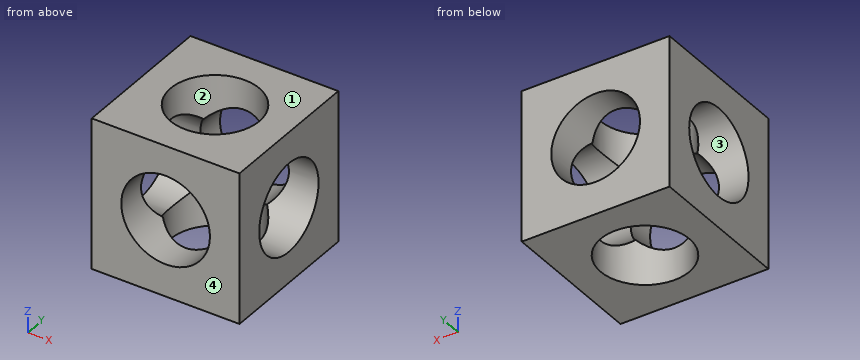
```python
from build123d import *

# Parameters (mm, degrees)
F0_W     = 126.93037
F0_H     = 126.93037
F0_R     = 38.1
F1_DEPTH = 129.5146
F2_R     = 38.1
F3_DEPTH = 129.5146
F4_R     = 38.1
F5_DEPTH = 129.5146


with BuildPart() as f1:
    # F0 (on Top) → F1 (new body)
    with BuildSketch(Plane.XY):
        Rectangle(F0_W, F0_H)
        Circle(F0_R, mode=Mode.SUBTRACT)
    extrude(amount=F1_DEPTH)

    # F2 (on face) → F3 (cut)
    with BuildSketch(Plane.XZ.offset(63.465185)):
        with Locations((0, 65.735653)):
            Circle(F2_R)
    extrude(amount=-F3_DEPTH, mode=Mode.SUBTRACT)

    # F4 (on face) → F5 (cut)
    with BuildSketch(Plane.YZ.offset(63.465185)):
        with Locations((0, 64.757302)):
            Circle(F4_R)
    extrude(amount=-F5_DEPTH, mode=Mode.SUBTRACT)


solid = f1.part
```
CAD build for the part. Positions are in the model's coordinates, mm. Face numbers are marked on the shaded views. Coordinates: 2 decimals unless noted, no trailing zeros. Order: outer loops, then holes, each group sorted by start corner. A loop starts at its lowest first (then second) coordinate and runs counter-clockwise, first axis right, second up.
(1) Pin check, flat tip, straight feed: pin 1 Ø6 at (x, y) = (-43.5, -49) entering from -Z. Stop position of the tip, or through.
Solution:
pin 1: stops at z = 0
(2) Saw through at D-D, the plane x = -55.5. Write the cut outline in (y, z), and give its area (3 significant figures).
Solution:
outline: (-63.47, 0) - (63.47, 0) - (63.47, 129.51) - (-63.47, 129.51) - close; hole circle Ø76.2 at (0, 64.76)
area: 11,900 mm2
(3) Mould opens along Y. For the marked faces 1, 2, 3 and 4 say: released by +Y, released by -Y, zero draft, split by the parting line, or undercut.
Solution:
face 1: zero draft
face 2: undercut
face 3: undercut
face 4: released by -Y
(4) Drill centre lines: L1, parallel to Y at x = 0, z = 12; L2, parallel to Z at x = 0, y = -48. Where is each one in solid material? Low to high.
Solution:
L1: y = -63.47 to -38.1, 38.1 to 63.47
L2: z = 0 to 27.64, 103.84 to 129.51
(5) Saw through at A-A, the plane y = 0. Write the cut outline in (x, z), and give its area (3 significant figures).
Solution:
outline: (-63.47, 0) - (-38.1, 0) - (-38.1, 26.66) - (-63.47, 26.66) - close; (-63.47, 102.86) - (-38.1, 102.86) - (-38.1, 129.51) - (-63.47, 129.51) - close; (38.1, 0) - (63.47, 0) - (63.47, 26.66) - (38.1, 26.66) - close; (38.1, 102.86) - (63.47, 102.86) - (63.47, 129.51) - (38.1, 129.51) - close
area: 2,700 mm2
(6) Saw through at B-B, the plane x = 0. Write the cut outline in (y, z).
Solution:
outline: (-63.47, 0) - (-38.1, 0) - (-38.1, 27.64) - (-63.47, 27.64) - close; (-63.47, 103.84) - (-38.1, 103.84) - (-38.1, 129.51) - (-63.47, 129.51) - close; (38.1, 0) - (63.47, 0) - (63.47, 27.64) - (38.1, 27.64) - close; (38.1, 103.84) - (63.47, 103.84) - (63.47, 129.51) - (38.1, 129.51) - close
(7) Saw through at C-C, the plane z = 12. Write the cut outline in (x, y), and give its area (3 significant figures).
Solution:
outline: (-63.47, -63.47) - (63.47, -63.47) - (63.47, 63.47) - (-63.47, 63.47) - close; hole circle Ø76.2 at (0, 0)
area: 11,600 mm2
